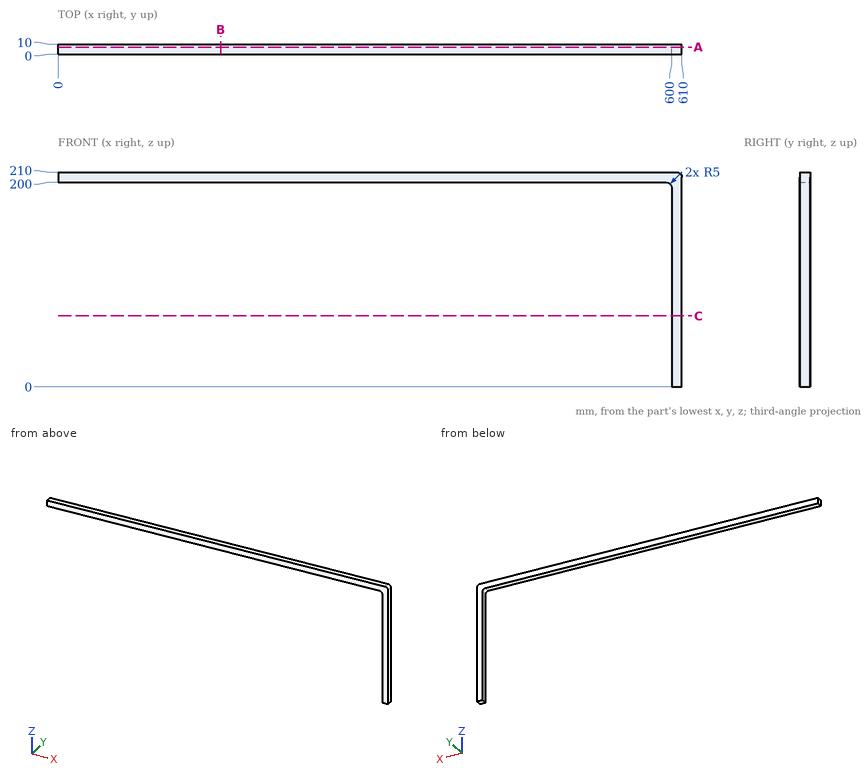
Geometry check sheet. Reference: drawing and pictorial views, mm from the part's lowest x, y, z. Coordinates: 2 decimals unless noted, no trailing zeros. Order: outer loops, then holes, each group sorted by start corner. A loop starts at its lowest first (then second) coordinate and runs counter-clockwise, first axis right, second up.
Item 1: Section check A-A (y = 7). Enter the section's corners in (x, z), plus the area to 3 significant figures.
Item 2: Scan lines: line 1 along Z through (x, y) = (454, 1); line 2 along X through (y, z) = (2, 43). Record each from-to range of solid material in increasing order.
Item 3: Section check C-C (z = 69.5). Enter the section's corners in (x, y).
Item 4: Depth check by flat-ended pin: pin 1 (1 mm diameter, centred on y = 7.5, z = 49, fed in from -X); pin 2 (5 mm diameter, centred on x = 335.5, y = 3, fed in from -Z). Enter the tip coordinate at first touch or a pass-through.
Item 5: Section check B-B (x = 159). Enter the section's corners in (y, z), plus the area to 3 significant figures.
Check sheet entries:
1. outline: (0, 200) - (595, 200) arc R5 cw to (600, 195) - (600, 0) - (610, 0) - (610, 205) arc R5 ccw to (605, 210) - (0, 210) - close
1. area: 8,100 mm2
2. line 1: z = 200 to 210
2. line 2: x = 600 to 610
3. outline: (600, 0) - (610, 0) - (610, 10) - (600, 10) - close
4. pin 1: stops at x = 600
4. pin 2: stops at z = 200
5. outline: (0, 200) - (10, 200) - (10, 210) - (0, 210) - close
5. area: 100 mm2
